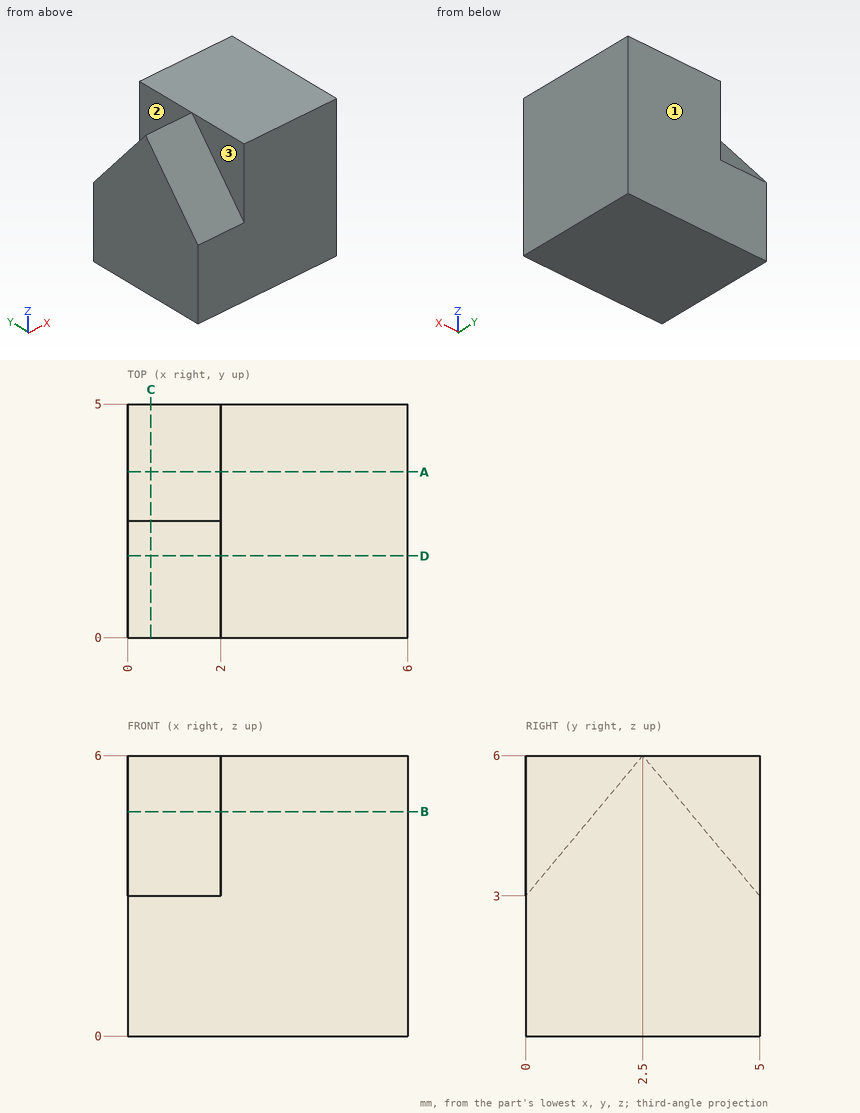
For this review, use the dimensioned drawing (mm, ordinates from the lowest corner) and the shaded views. A direction names the side the tool comes from. Round coordinates to 2 decimals unless told otherwise and drop trailing zeros. Write each loop counter-clockwise with the first axis right and the second up, starting at its lowest first coordinate (ties: lowest second). Pieces come first, ordered by that corner, then holes. Notation, with made-up numbers: M 78.5,-39.5 L 98.5,-39.5 A17 ccw 98.5,-10.5 Z; hole C 1,67 d8. An arc over 180 degrees is marked long. Write item = value, one per line. Start each with the question number.
(1) We need section C-C (x = 0.5). Give the boundary of the cut face in (y, z).
(2) For the marked faces 1, 2 and 3, list the 3-axis set-ups (+Z, -Z, +X, -X, +Y, -Y) from which the entire face can be reached by the end or side of a thin tool; tool diameter is ignored.
(3) We need section A-A (y = 3.55). Give the boundary of the cut face in (x, z), then the cut area to 3 significant figures.
(4) We need section D-D (y = 1.75). Give the boundary of the cut face in (x, z).
(5) We need section B-B (z = 4.8). Give the boundary of the cut face in (x, y).
(6) For line 1 along X through (y, z) = (0.8, 4.85); line 2 along Z through (x, y) = (1.7, 0.6); line 3 along Y through (x, z) = (1.35, 3.4), list the stretches that pass through material, from the lowest coordinate up.
Results found:
q1.outline = M 0,0 L 5,0 L 5,3 L 2.5,6 L 0,3 Z
q2.face_1 = +Z, -Z, +X, -X, +Y
q2.face_2 = +Z, -X, +Y
q2.face_3 = +Z, -X, -Y
q3.outline = M 0,0 L 6,0 L 6,6 L 2,6 L 2,4.74 L 0,4.74 Z
q3.area = 33.5 mm²
q4.outline = M 0,0 L 6,0 L 6,6 L 2,6 L 2,5.1 L 0,5.1 Z
q5.outline = M 0,1.5 L 2,1.5 L 2,0 L 6,0 L 6,5 L 2,5 L 2,3.5 L 0,3.5 Z
q6.line_1 = 2 to 6
q6.line_2 = 0 to 3.72
q6.line_3 = 0.33 to 4.67
